from build123d import *

# Parameters (mm, degrees)
F0_R     = 7
F1_DEPTH = 30
F3_D     = 4
F3_DEPTH = 10
F3_TIP   = 1.2017212381
F4_SIZE2 = 5.99999
F4_SIZE  = 29.99999


# Not quite as in the source:
# - a fillet or chamfer is up to 0.001 mm smaller than in the source, because OpenCascade refuses the exact size


with BuildPart() as f1:
    # F0 (on Top) → F1 (new body)
    with BuildSketch(Plane.XY):
        Circle(F0_R)
    extrude(amount=F1_DEPTH)

    # F3
    with Locations(Plane.XY.offset(30)):
        with Locations((0, 0)):
            Hole(F3_D / 2, depth=F3_DEPTH)
            with Locations((0, 0, -(F3_DEPTH + F3_TIP / 2))):  # 118° drill point
                Cone(0, F3_D / 2, F3_TIP, mode=Mode.SUBTRACT)

    # F4 (size 30 and 6 in the source; OpenCascade refuses exactly that, so slightly less here)
    f4_edges = [f1.edges().sort_by_distance(p)[0] for p in [
        (-7, 0, 0),
    ]]
    f4_side = f1.faces().sort_by_distance((-7, 0, 15))[0]
    chamfer(f4_edges, length=F4_SIZE, length2=F4_SIZE2, reference=f4_side)


solid = f1.part
Input: part model. Units: mm. Frame: model coordinates. A direction names the side the tool comes from. Round coordinates to 2 decimals unless told otherwise and drop trailing zeros. Write each loop counter-clockwise with the first axis right and the second up, starting at its lowest first coordinate (ties: lowest second). Pieces come first, ordered by that corner, then holes.
1) Cut plane B-B (z = 17). Return the cut outline in (x, y).
2) Contact query for flat-ended pins moving along their axis: P1, Ø2, axis at y = -4, z = 19.5, coming from the -X side; P2, Ø3, axis at x = -3.5, z = 12.5, coming from the -Y side; P3, Ø2, axis at y = -0.5, z = 9.5, coming from the -X side. Output: stop coordinate, or through.
3) Ray query, L1, parallel to Y at x = 1.75, z = 24.5; L2, parallel to X at y = 0, z = 26.5; L3, parallel to Y at x = 0, z = 26. Return the intervals inside material, ascending.
4) Reachability of faces 4 (the cylindrical face through (0, -2, 25)), 5 (the flat face through (0, 0, 0)) from +Z, -Z, +X, -X, +Y, -Y: full face, straight path, thin tool, end or side. Return the list, or none.
5) Draft query along Y for faces 1 (the flat face through (1, 2, 30)), 2 (the conical face through (-3.14, -2.41, 14.79)), 3 (the conical face through (-0.08, -0.34, 19.01)). Return one class per face: pulls with the +Y half, pulls with the -Y half, needs draft (parallel to the pull), parting line crosses it, or undercut.
6) Cut plane A-A (z = 28). Return the cut outline in (x, y).
7) Cut plane C-C (z = 9.25). Return the cut outline in (x, y).
Geometry says:
1. outline: circle Ø8.8 at (0, 0)
2. P1: stops at x = -3.91
2. P2: stops at y = -2.93
2. P3: stops at x = -3.08
3. L1: y = -5.63 to -0.97, 0.97 to 5.63
3. L2: x = -6.3 to -2, 2 to 6.3
3. L3: y = -6.2 to -2, 2 to 6.2
4. face 4: +Z
4. face 5: -Z, +X, -X, +Y, -Y
5. face 1: needs draft
5. face 2: parting line crosses it
5. face 3: undercut
6. outline: circle Ø13.2 at (0, 0); hole circle Ø4 at (0, 0)
7. outline: circle Ø5.7 at (0, 0)
